Design review of the part built by this model. Coordinates are the model's own, in mm. Coordinates: 2 decimals unless noted, no trailing zeros. Write each loop counter-clockwise with the first axis right and the second up, starting at its lowest first coordinate (ties: lowest second). Pieces come first, ordered by that corner, then holes. Notation, with made-up numbers: (-37, -24) - (-15, -24) arc R19 ccw to (-15, 7) - close; hole circle Ø8 at (2.25, -37.5). An arc over 180 degrees is marked (long way). Use a Markdown table: item, result.
from build123d import *

# Parameters (mm, degrees)
SKETCH1_W           = 96.52
SKETCH1_H           = 60.96
BOSS_EXTRUDE1_DEPTH = 0.9906
CUT_EXTRUDE1_REACH  = 2.991
SKETCH2_W           = 36.83
SKETCH2_H           = 10.16
SKETCH2_W_2         = 4.064
SKETCH2_H_2         = 26.035


with BuildPart() as part:
    # Sketch1 → Boss-Extrude1 (new body)
    with BuildSketch(Plane.XY):
        Rectangle(SKETCH1_W, SKETCH1_H)
    extrude(amount=BOSS_EXTRUDE1_DEPTH)

    # Sketch2 → Cut-Extrude1 (cut, up to next)
    with BuildSketch(Plane.XY.offset(0.9906), mode=Mode.PRIVATE) as cut_extrude1_sk1:
        with Locations((-26.035, -22.098)):
            Rectangle(SKETCH2_W, SKETCH2_H)
    cut_extrude1_tool1 = extrude(cut_extrude1_sk1.sketch, amount=-CUT_EXTRUDE1_REACH, mode=Mode.PRIVATE) & part.part
    add(cut_extrude1_tool1.solids().sort_by_distance((-26.035, -22.098, 0.9906))[0], mode=Mode.SUBTRACT)
    # Sketch2 → Cut-Extrude1 (cut, up to next)
    with BuildSketch(Plane.XY.offset(0.9906), mode=Mode.PRIVATE) as cut_extrude1_sk2:
        with Locations((15.748, 14.9225)):
            Rectangle(SKETCH2_W_2, SKETCH2_H_2)
    cut_extrude1_tool2 = extrude(cut_extrude1_sk2.sketch, amount=-CUT_EXTRUDE1_REACH, mode=Mode.PRIVATE) & part.part
    add(cut_extrude1_tool2.solids().sort_by_distance((15.748, 14.9225, 0.9906))[0], mode=Mode.SUBTRACT)


solid = part.part
(1) Take a section at A-A on y = -21. Write out the cut boundary in (x, z).
Determined:
| item | result |
|---|---|
| outline | (-48.26, 0) - (-44.45, 0) - (-44.45, 0.99) - (-48.26, 0.99) - close; (-7.62, 0) - (48.26, 0) - (48.26, 0.99) - (-7.62, 0.99) - close |
(2) For pin 1 (4 mm diameter, centred on x = -17.5, y = 23, fed in from -Z), flat-tipped, find the tip position at first contact; note if it passes through.
Determined:
| item | result |
|---|---|
| pin 1 | z = 0 |
(3) Take a section at B-B on x = 16.5. Write out the cut boundary in (y, z) (3 decimals), and give its area (3 significant figures).
Determined:
| item | result |
|---|---|
| outline | (-30.48, 0) - (1.905, 0) - (1.905, 0.991) - (-30.48, 0.991) - close; (27.94, 0) - (30.48, 0) - (30.48, 0.991) - (27.94, 0.991) - close |
| area | 34.6 mm2 |
(4) For L1, parallel to Y at x = -43, z = 0.75; L2, parallel to X at y = 11.5, z = 0.8; L3, parallel to X at y = -25, z = 0.35, list the stretches that pass through material, from the lowest coordinate up. Write a range as from..to.
Determined:
| item | result |
|---|---|
| L1 | -30.48..-27.18, -17.02..30.48 |
| L2 | -48.26..13.72, 17.78..48.26 |
| L3 | -48.26..-44.45, -7.62..48.26 |
(5) Take a section at C-C on z = 0.25. Write out the cut boundary in (x, y) (3 decimals).
Determined:
| item | result |
|---|---|
| outline | (-48.26, -30.48) - (48.26, -30.48) - (48.26, 30.48) - (-48.26, 30.48) - close; hole (-44.45, -27.178) - (-7.62, -27.178) - (-7.62, -17.018) - (-44.45, -17.018) - close; hole (13.716, 1.905) - (17.78, 1.905) - (17.78, 27.94) - (13.716, 27.94) - close |
